Drawing for the job (mm, zero at the part's lowest x, y, z). Give positions to 0.01 mm unless a question says otherwise; leave off trailing zeros. Loops run counter-clockwise (first coordinate to the right, second up) from the corner with the lowest first, then second, coordinate; pieces in that order, holes last. Notation, with made-up numbers: (53.25, 11.5) -> (75.25, 11.5) arc R25 ccw to (75.25, 29.5) -> close; hole circle Ø10 at (2, -7.5). An arc over 180 degrees is marked (long way). Use CSV: the item, a comma, the result in double quotes. Start each with the question number.
(1) Drill centre lines: probe 1 along Y at (x, z) = (26.67, 0.9); probe 2 along X at (y, z) = (10, 0.65); probe 3 along Y at (x, z) = (5.5, 1.05). Where is each one in solid material? Low to high.
(2) Cut at B-B on y = 20.32. Write the cut outline in (x, z).
(3) Cut at D-D on x = 9. Write the cut outline in (y, z), then the cut area to 3 significant figures.
(4) Cut at A-A on x = 26.67. Write the cut outline in (y, z).
(5) Cut at C-C on z = 0.7. State how many separate pieces and enclosed holes the cut face has, then the cut area to 3 significant figures.
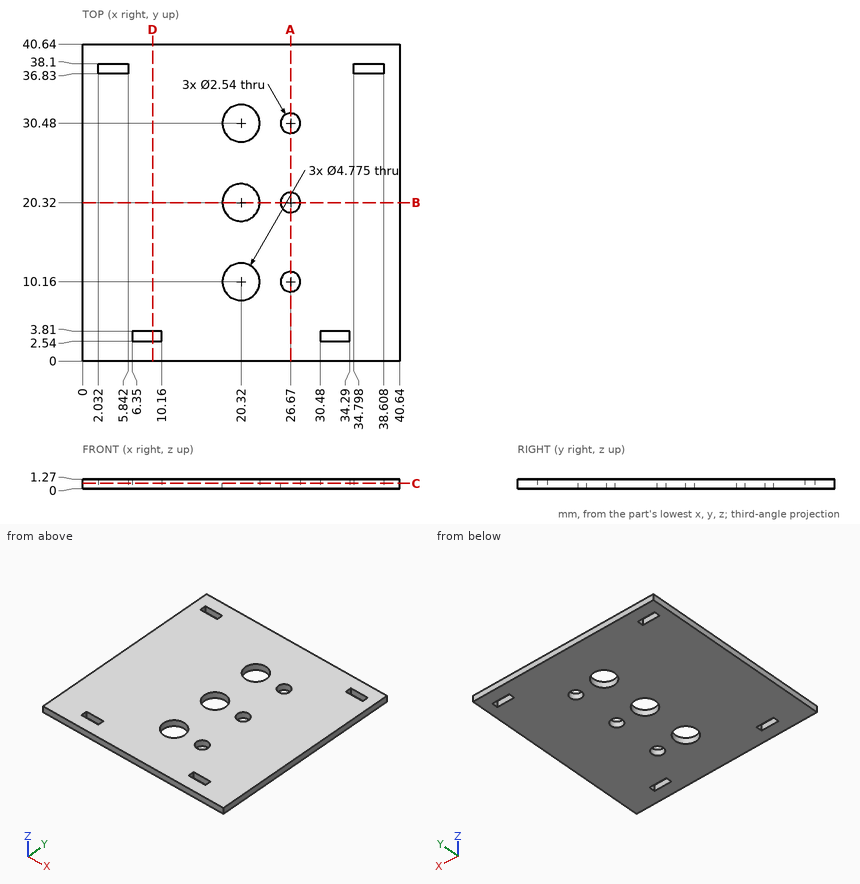
Check result:
1,probe 1,"0 to 8.89, 11.43 to 19.05, 21.59 to 29.21, 31.75 to 40.64"
1,probe 2,"0 to 17.94, 22.7 to 25.41, 27.93 to 40.64"
1,probe 3,"0 to 36.83, 38.1 to 40.64"
2,outline,"(0, 0) -> (17.93, 0) -> (17.93, 1.27) -> (0, 1.27) -> close; (22.71, 0) -> (25.4, 0) -> (25.4, 1.27) -> (22.71, 1.27) -> close; (27.94, 0) -> (40.64, 0) -> (40.64, 1.27) -> (27.94, 1.27) -> close"
3,outline,"(0, 0) -> (2.54, 0) -> (2.54, 1.27) -> (0, 1.27) -> close; (3.81, 0) -> (40.64, 0) -> (40.64, 1.27) -> (3.81, 1.27) -> close"
3,area,"50.0 mm²"
4,outline,"(0, 0) -> (8.89, 0) -> (8.89, 1.27) -> (0, 1.27) -> close; (11.43, 0) -> (19.05, 0) -> (19.05, 1.27) -> (11.43, 1.27) -> close; (21.59, 0) -> (29.21, 0) -> (29.21, 1.27) -> (21.59, 1.27) -> close; (31.75, 0) -> (40.64, 0) -> (40.64, 1.27) -> (31.75, 1.27) -> close"
5,separate pieces,"1"
5,enclosed holes,"10"
5,area,"1,560 mm²"
